Verification items for the finished model (mm, model axes). Face numbers are marked on the shaded views. Round coordinates to 2 decimals unless told otherwise and drop trailing zeros. Order: outer loops, then holes, each group sorted by start corner. A loop starts at its lowest first (then second) coordinate and runs counter-clockwise, first axis right, second up. Notation, with made-up numbers: (-37, -17.5) -> (-26, -17.5) arc R10 cw to (-26, -12.5) -> close; hole circle Ø2 at (-37, 82.5). An arc over 180 degrees is marked (long way). Put each result on its own line as item: value.
```python
from build123d import *

# Parameters (mm, degrees)
SKETCH1_W             = 180
SKETCH1_H             = 180
BOSS_EXTRUDE1_DEPTH   = 5
SKETCH2_R             = 20
BOSS_EXTRUDE2_DEPTH   = 95
BOSS_EXTRUDE3_START   = -5
BOSS_EXTRUDE3_DEPTH   = 5
CUT_EXTRUDE1_REACH    = 182.278
SKETCH4_R             = 10
BODY_MOVE_COPY1_ANGLE = 90


with BuildPart() as part:
    # Sketch1 → Boss-Extrude1 (new body)
    with BuildSketch(Plane(origin=(0, 0, 0), x_dir=(1, 0, 0), z_dir=(0, 1, 0))):
        Rectangle(SKETCH1_W, SKETCH1_H)
    extrude(amount=BOSS_EXTRUDE1_DEPTH)

    # Sketch2 → Boss-Extrude2 (add)
    with BuildSketch(Plane(origin=(0, 5, 0), x_dir=(1, 0, 0), z_dir=(0, 1, 0))):
        with Locations(Location((0, 0, 0), (0, 0, 270))):
            Circle(SKETCH2_R)
    extrude(amount=BOSS_EXTRUDE2_DEPTH)

    # Sketch3 → Boss-Extrude3 (add)
    with BuildSketch(Plane(origin=(0, 100, 0), x_dir=(1, 0, 0), z_dir=(0, 1, 0)).offset(BOSS_EXTRUDE3_START)):
        with BuildLine():
            Line((0, 20), (100, 20))
            ThreePointArc((100, 20), (120, 0), (100, -20))
            Line((100, -20), (0, -20))
            ThreePointArc((0, -20), (-20, 0), (0, 20))
        make_face()
    extrude(amount=BOSS_EXTRUDE3_DEPTH)

    # Sketch4 → Cut-Extrude1 (cut, up to next)
    with BuildSketch(Plane(origin=(0, 100, 0), x_dir=(1, 0, 0), z_dir=(0, 1, 0)), mode=Mode.PRIVATE) as cut_extrude1_sk1:
        with Locations(Location((95, 0, 0), (0, 0, 270))):
            Circle(SKETCH4_R)
    cut_extrude1_tool1 = extrude(cut_extrude1_sk1.sketch, amount=-CUT_EXTRUDE1_REACH, mode=Mode.PRIVATE) & part.part
    add(cut_extrude1_tool1.solids().sort_by_distance((95, 100, 0))[0], mode=Mode.SUBTRACT)


with BuildPart() as part_1:
    # Body-Move/Copy1: moved
    add(part.part.rotate(Axis((0, 0, 0), (1, 0, 0)), BODY_MOVE_COPY1_ANGLE))


solid = part_1.part
```
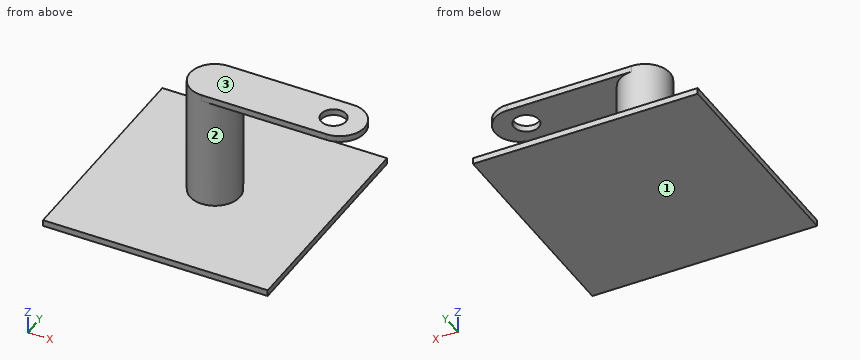
Item 1: Sectioned sample at A-A, the plane x = 95. Record the boundary of the cut face in (y, z).
Geometry check:
outline: (-20, 95) -> (-10, 95) -> (-10, 100) -> (-20, 100) -> close; (10, 95) -> (20, 95) -> (20, 100) -> (10, 100) -> close
Item 2: Sectioned sample at B-B, the plane y = 0. Record the boundary of the cut face in (x, z).
Geometry check:
outline: (-90, 0) -> (90, 0) -> (90, 5) -> (20, 5) -> (20, 95) -> (85, 95) -> (85, 100) -> (-20, 100) -> (-20, 5) -> (-90, 5) -> close; (105, 95) -> (120, 95) -> (120, 100) -> (105, 100) -> close
Item 3: Material ranges on line 1 along X through (y, z) = (0, 98.9); line 2 along Z through (x, y) = (62, 9); line 3 along Z through (x, y) = (-7.5, 26), recorded low to high.
Geometry check:
line 1: -20 to 85, 105 to 120
line 2: 0 to 5, 95 to 100
line 3: 0 to 5
Item 4: Release check for a two-part mould opening along Z. For the marked faces 1, 2 and 3 record: pulls with the +Z half, pulls with the -Z half, needs draft (parallel to the pull), parting line crosses it, or undercut.
Geometry check:
face 1: pulls with the -Z half
face 2: undercut
face 3: pulls with the +Z half
Item 5: Depth check by flat-ended pin: pin 1 Ø2.5 at (x, z) = (42.5, 98) entering from +Y; pin 2 Ø4 at (y, z) = (-8, 2.5) entering from +X; pin 3 Ø4 at (x, z) = (43.5, 96.5) entering from -Y. Enter the tip coordinate at first touch or a pass-through.
Geometry check:
pin 1: y = 20
pin 2: x = 90
pin 3: y = -20
Item 6: Sectioned sample at D-D, the plane y = 46.5. Record the boundary of the cut face in (x, z), then the cut area to 3 significant figures.
Geometry check:
outline: (-90, 0) -> (90, 0) -> (90, 5) -> (-90, 5) -> close
area: 900 mm2
Item 7: Sectioned sample at C-C, the plane x = 36. Record the boundary of the cut face in (y, z), then the cut area to 3 significant figures.
Geometry check:
outline: (-90, 0) -> (90, 0) -> (90, 5) -> (-90, 5) -> close; (-20, 95) -> (20, 95) -> (20, 100) -> (-20, 100) -> close
area: 1,100 mm2
